Autodesk Inventor part; units mm, degrees
sketch "Sketch1" plane through (0, 0, 0) normal (0, 0, 1) x (1, 0, 0)
  line L0 (-15, 0) -> (15, 0)
  line L1 (-15, 5) -> (-15, 0)
  line L2 (15, 5) -> (15, 0)
  line L3 (15, 5) -> (7.5, 5)
  line L4 (-15, 5) -> (-7.5, 5)
  line L5 (-7.5, 5) -> (-7.5, 10)
  line L6 (7.5, 5) -> (7.5, 10)
  line L7 (7.5, 10) -> (-7.5, 10)
  point P0 (0, 0)
  point P1 (0, 0)
  dimension "d0" = 30
  dimension "d1" = 5
  dimension "d2" = 15
extrude "Extrusion1" add sketch "Sketch1" along normal blind 19
sketch "Sketch2" plane through (-15, 5, 0) normal (0, 1, 0) x (1, 0, 0)
  circle A0 centre (3.75, -9.5) radius 3.1
  line L0 (0, 0) -> (30, 0)
  line L1 (0, 0) -> (0, -19)
  line L2 (0, 0) -> (0, -19)
  line L3 (0, 0) -> (7.5, 0)
  point P0 (15, 0)
  point P1 (0, -9.5)
  point P2 (3.75, 0)
  dimension "d5" = 6.2
extrude "Extrusion2" cut sketch "Sketch2" against normal through all
mirror "Mirror1" about plane through (0, 0, 0) normal (1, 0, 0) of "Extrusion2"
sketch "Sketch3" plane through (0, 0, 19) normal (0, 0, 1) x (1, 0, 0)
  circle A0 centre (0, 5) radius 3.25
  line L0 (-15, 0) -> (15, 0)
  point P0 (0, 0)
  point P1 (0, 0)
  point P2 (-7.5, 5)
  dimension "d9" = 6.5
extrude "Extrusion3" cut sketch "Sketch3" against normal through all
sketch "Sketch4" plane through (-7.5, 10, 0) normal (0, 1, 0) x (1, 0, 0)
  circle A0 centre (7.5, -9.5) radius 3.1
  line L0 (15, 0) -> (0, 0)
  line L1 (0, 0) -> (0, -19)
  point P0 (7.5, 0)
  point P1 (7.5, 0)
  point P2 (0, -9.5)
  dimension "d12" = 6.2
extrude "Extrusion4" cut sketch "Sketch4" against normal up to next
ref_plane "Work Plane1" through (0, 0, 9.5) normal (0, 0, -1) x (-1, 0, 0)
properties part number "suporte_veio_001_001" material "Aluminum 6061"
Read the model definition and answer for the solid it produces. Units are mm, in the model's axes. A direction names the side the tool comes from. Coordinates: 2 decimals unless noted, no trailing zeros. Write each loop counter-clockwise with the first axis right and the second up, starting at its lowest first coordinate (ties: lowest second). Pieces come first, ordered by that corner, then holes. Notation, with made-up numbers: (-13.75, 14) -> (-3.75, 14) arc R5 cw to (-3.75, 20) -> close; hole circle Ø3 at (0, 21.25). An arc over 180 degrees is marked (long way). Answer as a JSON object with one key per item and string values.
Q1. Determine the mould class of faces 1 (the cylindrical face through (-0.705, 1.827, 9.633)), 2 (the flat face through (7.5, 7, 9)), 3 (the flat face through (3.4, 10, 9.4)), 4 (the flat face through (-15, 3, 9)) for opening direction X: pulls with the +X half, pulls with the -X half, needs draft (parallel to the pull), parting line crosses it, or undercut.
The answers:
{"face 1": "undercut", "face 2": "pulls with the +X half", "face 3": "needs draft", "face 4": "pulls with the -X half"}
Q2. A tool of negligible diameter and unlimited length cuts with its end or side. For faces 5 (the cylindrical face through (2.864, 8.462, 10.687)), 6 (the flat face through (-4, 4, 19)), 7 (the flat face through (9, 5, 7)), 8 (the flat face through (15, 3, 9)), 9 (the flat face through (-7.5, 7, 9)), from which of +Z, -Z, +X, -X, +Y, -Y can it reach the whole face along a straight path? Write none if from no direction.
The answers:
{"face 5": "+Y", "face 6": "+Z, +X, -X, +Y, -Y", "face 7": "+Z, -Z, +X, +Y", "face 8": "+Z, -Z, +X, +Y, -Y", "face 9": "+Z, -Z, -X, +Y"}
Q3. The part is cut by section C-C on y = 3.5. Give the vertices of the cut face in (x, z).
The answers:
{"outline": "(-15, 0) -> (-2.88, 0) -> (-2.88, 19) -> (-15, 19) -> close; (2.88, 0) -> (15, 0) -> (15, 19) -> (2.88, 19) -> close; hole circle Ø6.2 at (-11.25, 9.5); hole circle Ø6.2 at (11.25, 9.5)"}
Q4. The part is cut by section A-A on z = 9.5. Give the vertices of the cut face in (x, y).
The answers:
{"outline": "(-15, 0) -> (-14.35, 0) -> (-14.35, 5) -> (-15, 5) -> close; (-8.15, 0) -> (8.15, 0) -> (8.15, 5) -> (7.5, 5) -> (7.5, 10) -> (3.1, 10) -> (3.1, 5.98) arc R3.25 cw (long way) to (-3.1, 5.98) -> (-3.1, 10) -> (-7.5, 10) -> (-7.5, 5) -> (-8.15, 5) -> close; (14.35, 0) -> (15, 0) -> (15, 5) -> (14.35, 5) -> close"}
Q5. Consider line 1 (Y direction, x = 0, z = 5); line 2 (X direction, y = 9, z = 9.5); line 3 (Z direction, x = 0, y = 8.8). Determine where each line is inside the solid, lowest interval first. Write a range as [from, to].
The answers:
{"line 1": "y = [0, 1.75], [8.25, 10]", "line 2": "x = [-7.5, -3.1], [3.1, 7.5]", "line 3": "z = [0, 6.4], [12.6, 19]"}
Q6. Flat-ended cylindrical pins translate along their axes: pin 1 Ø1.5 at (y, z) = (8.5, 9.5) entering from +X; pin 2 Ø7 at (x, z) = (11.25, 9.5) entering from -Y; pin 3 Ø5 at (y, z) = (8, 10) entering from -X; pin 4 Ø4 at (x, z) = (10, 8) entering from +Y. Find the tip coordinate at first contact, or state that the pin passes through.
The answers:
{"pin 1": "stops at x = 7.5", "pin 2": "stops at y = 0", "pin 3": "stops at x = -7.5", "pin 4": "stops at y = 5"}
Q7. The part is cut by section D-D on y = 1. Give the vertices of the cut face in (x, z), then the cut area to 3 significant figures.
The answers:
{"outline": "(-15, 0) -> (15, 0) -> (15, 19) -> (-15, 19) -> close; hole circle Ø6.2 at (-11.25, 9.5); hole circle Ø6.2 at (11.25, 9.5)", "area": "510 mm2"}
Q8. The part is cut by section B-B on x = -11.25. Give the vertices of the cut face in (y, z), then the cut area to 3 significant figures.
The answers:
{"outline": "(0, 0) -> (5, 0) -> (5, 6.4) -> (0, 6.4) -> close; (0, 12.6) -> (5, 12.6) -> (5, 19) -> (0, 19) -> close", "area": "64.0 mm2"}
